CAD build for the part. Positions are in the model's coordinates, mm. A direction names the side the tool comes from. Coordinates: 2 decimals unless noted, no trailing zeros. Order: outer loops, then holes, each group sorted by start corner. A loop starts at its lowest first (then second) coordinate and runs counter-clockwise, first axis right, second up. Notation, with made-up numbers: (-29.75, 0.5) -> (-23.75, 0.5) arc R15 ccw to (-23.75, 29.5) -> close; hole circle Ø9 at (75.25, 14.5). An arc over 180 degrees is marked (long way). Use one line per item in the form item = value. Start each with the question number.
from build123d import *

# Parameters (mm, degrees)
BOSS_EXTRUDE1_DEPTH = 16
SKETCH2_R           = 2
CUT_EXTRUDE1_DEPTH  = 16
SKETCH3_R           = 2
BOSS_EXTRUDE2_DEPTH = 2
SKETCH4_R           = 4.5
CUT_EXTRUDE2_DEPTH  = 2


with BuildPart() as part:
    # Sketch1 → Boss-Extrude1 (new body)
    with BuildSketch(Plane(origin=(0, 0, 0), x_dir=(1, 0, 0), z_dir=(0, 1, 0))):
        Polygon((-4.620689655, 26), (-4.620689655, -7.5), (15.379310345, -7.5), (15.379310345, -5.5), (-2.620689655, -5.5), (-2.620689655, 26), align=None)
    extrude(amount=BOSS_EXTRUDE1_DEPTH)

    # Sketch2 → Cut-Extrude1 (cut)
    with BuildSketch(Plane.XY.offset(7.5)):
        with Locations((0.379310345, 8)):
            Circle(SKETCH2_R)
        with Locations((10.379310345, 8)):
            Circle(SKETCH2_R)
    extrude(amount=-CUT_EXTRUDE1_DEPTH, mode=Mode.SUBTRACT)

    # Sketch3 → Boss-Extrude2 (add)
    # profile 1 of 2: a face of its own
    with BuildSketch(Plane.ZY.offset(4.620689655)):
        with BuildLine():
            Line((-16, 16), (-8, 16))
            Line((-8, 16), (-8, 25.5))
            ThreePointArc((-8, 25.5), (-12, 29.5), (-16, 25.5))
            Line((-16, 25.5), (-16, 16))
        make_face()
        with Locations((-12, 25.5)):
            Circle(SKETCH3_R, mode=Mode.SUBTRACT)
    # profile 2 of 2: a face of its own
    with BuildSketch(Plane.ZY.offset(4.620689655)):
        with BuildLine():
            Line((-16, 0), (-8, 0))
            Line((-8, 0), (-8, -9.5))
            ThreePointArc((-8, -9.5), (-12, -13.5), (-16, -9.5))
            Line((-16, -9.5), (-16, 0))
        make_face()
        with Locations((-12, -9.5)):
            Circle(SKETCH3_R, mode=Mode.SUBTRACT)
    extrude(amount=-BOSS_EXTRUDE2_DEPTH)

    # Sketch4 → Cut-Extrude2 (cut)
    with BuildSketch(Plane.ZY.offset(4.620689655)):
        with Locations((-4, 8)):
            Circle(SKETCH4_R)
    extrude(amount=-CUT_EXTRUDE2_DEPTH, mode=Mode.SUBTRACT)


solid = part.part
1) Probe L1, parallel to Y at x = -3.8, z = -12; L2, parallel to X at y = 4, z = -9; L3, parallel to Z at x = 9, y = 13. List the from-to ranges inside material, lowest first.
2) Cut at C-C on z = -12. Give the cut face in (x, y).
3) Two-plate mould, pull along Z, no slides. Class faces 6 (the face through (-3.6, 24.3, -13.6)), 7 (the face through (-3.6, 29.5, -11.9)), 8 (the face through (-4.621, 8, -9)): released by +Z, released by -Z, zero draft, split by the parting line, or undercut.
4) Cut at B-B on y = 8. Give the cut face in (x, z), then the cut area to 3 significant figures.
5) 3-axis set-ups, long thin cutter, end or side, ignore diameter. For faces 1 (the face through (-4, -5, -16)), 2 (the face through (-4, -5, -8)), 3 (the face through (-4, 21, -16)), 4 (the face through (-2.621, 8, -10)), 5 (the face through (-4, 21, -8)): which of +Z, -Z, +X, -X, +Y, -Y reach the whole face in a straight line?
6) Drop flat-ended pins along their axis: P1, Ø8, axis at y = 16, z = -6, coming from the +X side; P2, Ø1.6, axis at x = -4, y = 21, coming from the +Z side; P3, Ø8, axis at x = -1, y = 24.5, coming from the -Z side; P4, Ø6, axis at x = 1, z = -14, coming from the +Y side. Give the stop position or say it passes through.
7) Cut at A-A on z = -4. Give the cut face in (x, y).
8) Cut at D-D on x = 11. Give the cut face in (y, z), then the cut area to 3 significant figures.
Values follow:
q1.L1 = -13.5 to -11.5, -7.5 to 23.5, 27.5 to 29.5
q1.L2 = -4.62 to -2.62
q1.L3 = 5.5 to 7.5
q2.outline = (-4.62, -13.5) -> (-2.62, -13.5) -> (-2.62, -11.5) -> (-4.62, -11.5) -> close; (-4.62, -7.5) -> (-2.62, -7.5) -> (-2.62, 23.5) -> (-4.62, 23.5) -> close; (-4.62, 27.5) -> (-2.62, 27.5) -> (-2.62, 29.5) -> (-4.62, 29.5) -> close
q3.face_6 = undercut
q3.face_7 = split by the parting line
q3.face_8 = zero draft
q4.outline = (-4.62, -26) -> (-2.62, -26) -> (-2.62, -8.5) -> (-4.62, -8.5) -> close; (-4.62, 0.5) -> (-2.62, 0.5) -> (-2.62, 5.5) -> (-1.62, 5.5) -> (-1.62, 7.5) -> (-4.62, 7.5) -> close; (2.38, 5.5) -> (8.38, 5.5) -> (8.38, 7.5) -> (2.38, 7.5) -> close; (12.38, 5.5) -> (15.38, 5.5) -> (15.38, 7.5) -> (12.38, 7.5) -> close
q4.area = 69.0 mm^2
q5.face_1 = -Z, +X, -X, -Y
q5.face_2 = +Z, +X, -X, -Y
q5.face_3 = -Z, +X, -X, +Y
q5.face_4 = -Z, +X, +Y, -Y
q5.face_5 = +Z, +X, -X, +Y
q6.P1 = -2.62
q6.P2 = -8
q6.P3 = -16
q6.P4 = through
q7.outline = (-4.62, 0) -> (-2.62, 0) -> (-2.62, 3.5) -> (-4.62, 3.5) -> close; (-4.62, 12.5) -> (-2.62, 12.5) -> (-2.62, 16) -> (-4.62, 16) -> close
q8.outline = (0, 5.5) -> (6.1, 5.5) -> (6.1, 7.5) -> (0, 7.5) -> close; (9.9, 5.5) -> (16, 5.5) -> (16, 7.5) -> (9.9, 7.5) -> close
q8.area = 24.4 mm^2
